Source: CAD feature listing. Evaluate the final solid. Frame: model axes, mm. A direction names the side the tool comes from. Round coordinates to 2 decimals unless told otherwise and drop trailing zeros. Write each loop counter-clockwise with the first axis right and the second up, starting at its lowest first coordinate (ties: lowest second). Pieces come first, ordered by that corner, then holes.
from build123d import *

# Parameters (mm, degrees)
CHANFREIN1_SIZE = 0.5
CONG_1_R        = 0.3


with BuildPart() as part:
    # Esquisse1 → Révol.-Mince2 (revolve)
    with BuildSketch(Plane.XY, mode=Mode.PRIVATE) as r_vol_mince2_sk:
        Polygon((0, 0), (0, 16), (8, 16), (8, 15), (1, 15), (1, 0), align=None)
    revolve(r_vol_mince2_sk.sketch.rotate(Axis((-7.892655367, 0, 0), (1, 0, 0)), 90), axis=Axis((-7.892655367, 0, 0), (1, 0, 0)))

    # Chanfrein1
    chanfrein1_edges = [part.edges().sort_by_distance(p)[0] for p in [
        (8, 0, -16),
    ]]
    chamfer(chanfrein1_edges, length=CHANFREIN1_SIZE)

    # Congé1
    cong_1_edges = [part.edges().sort_by_distance(p)[0] for p in [
        (0, 0, -16),
    ]]
    fillet(cong_1_edges, radius=CONG_1_R)


solid = part.part
1) Section query C-C on x = 3. Return the cut outline in (y, z).
Taken from the geometry:
outline: circle Ø32 at (0, 0); hole circle Ø30 at (0, 0)
2) Section query A-A on y = 0. Return the cut outline in (x, z).
Taken from the geometry:
outline: (0, -15.7) arc R0.3 ccw to (0.3, -16) - (7.5, -16) - (8, -15.5) - (8, -15) - (1, -15) - (1, 15) - (8, 15) - (8, 15.5) - (7.5, 16) - (0.3, 16) arc R0.3 ccw to (0, 15.7) - close
3) Material intervals for line 1 (Y direction, x = 5.5, z = 0); line 2 (X direction, y = -7, z = 2.5); line 3 (Y direction, x = 7, z = -6), sorted ascending.
Taken from the geometry:
line 1: y = -16 to -15, 15 to 16
line 2: x = 0 to 1
line 3: y = -14.83 to -13.75, 13.75 to 14.83
4) Pull-direction query (Y, two-part tool) for faces 3 (the face through (8, -13, -8)), 4 (the face through (3.95, 15.62, -3.47)), 5 (the face through (1, 0, 0)); classes: released by +Y, released by -Y, zero draft, split by the parting line, or undercut.
Taken from the geometry:
face 3: zero draft
face 4: split by the parting line
face 5: undercut
5) Contact query for flat-ended pins moving along their axis: P1, Ø2, axis at x = 6, z = 3, coming from the -Y side; P2, Ø1.5, axis at x = 4, z = 6.5, coming from the +Y side; P3, Ø6, axis at y = 2, z = 6, coming from the -X side; P4, Ø18, axis at y = 0, z = 0, coming from the +X side. Output: stop coordinate, or through.
Taken from the geometry:
P1: stops at y = -15.87
P2: stops at y = 14.93
P3: stops at x = 0
P4: stops at x = 1
6) Reachability of faces 1 (the face through (4.45, -12.65, 8.06)), 2 (the face through (0, 0, 0)) from +Z, -Z, +X, -X, +Y, -Y: full face, straight path, thin tool, end or side. Return the list, or none.
Taken from the geometry:
face 1: +X
face 2: +Z, -Z, -X, +Y, -Y
